For this review, take the finished solid that the model builds, in its own axes (mm). A direction names the side the tool comes from. Give positions to 0.01 mm unless a question says otherwise; leave off trailing zeros. Write each loop counter-clockwise with the first axis right and the second up, starting at its lowest first coordinate (ties: lowest second). Pieces come first, ordered by that corner, then holes.
Q1. We need section D-D (y = -4.25). Write out the cut boundary in (x, z), then the cut area to 3 significant figures.
Q2. We need section C-C (z = -0.5). Write out the cut boundary in (x, y).
Q3. Machinability: for faces 1 (the flat face through (-21, -0.5, 0)), 2 (the flat face through (0, 0, 0)), 3 (the flat face through (-25.5, 3, 0)), 4 (the flat face through (-21, 3, 1.5)), 5 (the flat face through (-21, 7, 0)), which of the approach directions +Z, -Z, +X, -X, +Y, -Y give a long, thin tool a straight path to every point of the face, cutting with its end or side? Answer none if there is none.
Q4. For line 1 (Z direction, x = 3, y = -2.75); line 2 (Y direction, x = -23, z = 1.25); line 3 (X direction, y = 3.5, z = -1), list the stretches that pass through material, from the lowest coordinate up.
Q5. Insertion check: P1, Ø2, axis at y = 3.5, z = 3.5, coming from the -X side; P2, Ø5, axis at x = 10, y = -5.5, coming from the -Z side; P3, Ø2.5, axis at x = -21.5, z = 0.5, coming from the +Y side. Each pin has a flat end and moves straight along its axis. Give the tip position at first contact, or say it passes through.
Q6. We need section A-A (y = 0.25). Write out the cut boundary in (x, z).
Q7. We need section B-B (x = -22). Write out the cut boundary in (y, z).
```python
from build123d import *

# Parameters (mm, degrees)
F1_DEPTH = 6
F0_W     = 8.25
F0_H     = 7.5
F2_DEPTH = 1.5
F3_SIZE2 = 5
F3_SIZE  = 1.25
F4_SIZE2 = 2.5
F4_SIZE  = 5


with BuildPart() as f1:
    # F0 (on Top) → F1 (new body)
    with BuildSketch(Plane.XY):
        Polygon((17.25, 9), (-17.25, 9), (-17.25, 7), (-17.25, -0.5), (-17.25, -9), (17.25, -9), align=None)
    extrude(amount=F1_DEPTH)

    # F0 (on Top) → F2 (join, symmetric)
    with BuildSketch(Plane.XY):
        with Locations((-21.375, 3.25)):
            Rectangle(F0_W, F0_H)
    extrude(amount=F2_DEPTH, both=True)

    # F3
    f3_edges = [f1.edges().sort_by_distance(p)[0] for p in [
        (0, -9, 6),
        (0, 9, 6),
    ]]
    f3_side = f1.faces().sort_by_distance((0, 0, 6))[0]
    chamfer(f3_edges, length=F3_SIZE, length2=F3_SIZE2, reference=f3_side)

    # F4
    f4_edges = [f1.edges().sort_by_distance(p)[0] for p in [
        (17.25, 0, 6),
    ]]
    f4_side = f1.faces().sort_by_distance((17.25, 0, 2.9181))[0]
    chamfer(f4_edges, length=F4_SIZE, length2=F4_SIZE2, reference=f4_side)


solid = f1.part
```
Computed:
1. outline: (-17.25, 0) - (17.25, 0) - (17.25, 1) - (14.75, 6) - (-17.25, 6) - close
1. area: 201 mm2
2. outline: (-25.5, -0.5) - (-17.25, -0.5) - (-17.25, 7) - (-25.5, 7) - close
3. face 1: +Z, -Z, -X, -Y
3. face 2: -Z, +X, +Y, -Y
3. face 3: +Z, -Z, -X, +Y, -Y
3. face 4: +Z, -X, +Y, -Y
3. face 5: +Z, -Z, -X, +Y
4. line 1: z = 0 to 6
4. line 2: y = -0.5 to 7
4. line 3: x = -25.5 to -17.25
5. P1: stops at x = -17.25
5. P2: stops at z = 0
5. P3: stops at y = 7
6. outline: (-25.5, -1.5) - (-17.25, -1.5) - (-17.25, 0) - (17.25, 0) - (17.25, 1) - (14.75, 6) - (-17.25, 6) - (-17.25, 1.5) - (-25.5, 1.5) - close
7. outline: (-0.5, -1.5) - (7, -1.5) - (7, 1.5) - (-0.5, 1.5) - close
